Autodesk Inventor part; units mm, degrees
ref_plane "YZ Plane" through (0, 0, 0) normal (1, 0, 0) x (0, 1, 0)
ref_plane "XZ Plane" through (0, 0, 0) normal (0, 1, 0) x (-1, 0, 0)
ref_plane "XY Plane" through (0, 0, 0) normal (0, 0, 1) x (1, 0, 0)
sketch "Sketch_1" plane through (0, 0, 0) normal (0, 0, 1) x (1, 0, 0)
  line L0 (5, 0) -> (-0.8, 0)
  line L1 (-0.8, 0) -> (-0.8, 2)
  line L2 (-0.8, 2) -> (-0.2226, 3)
  line L3 (-0.2226, 3) -> (0, 3)
  line L4 (0, 3) -> (0, 1.4467)
  arc A0 (0, 1.4467) -> (0.1, 1.3467) centre (0.1, 1.4467) ccw
  line L5 (0.1, 1.3467) -> (0.9, 1.3467)
  line L6 (0.9, 1.3467) -> (1.4, 1.5)
  line L7 (1.4, 1.5) -> (4.6935, 1.5)
  line L8 (4.6935, 1.5) -> (5, 1.1935)
  line L9 (5, 1.1935) -> (5, 0)
  line L10 (5, 0) -> (-0.8, 0)
revolve "Revolution1" add sketch "Sketch_1" angle 360 about axis through (5, 0, 0) along (1, 0, 0)
thread "Thread1"
sketch "Sketch2" plane through (-0.8, 0, 0) normal (-1, 0, 0) x (0, 0, 1)
  point P0 (0, 0)
hole "Hole1" at (-0.8, 0, 0) direction (1, 0, 0) diameter 1.5 depth 2 tip angle 120
sketch "Sketch_3" plane through (-0.8, 0, 0) normal (1, 0, 0) x (0, 0, -1)
  line L0 (-0.75, -0.433) -> (0, -0.866)
  line L1 (0, -0.866) -> (0.75, -0.433)
  line L2 (0.75, -0.433) -> (0.75, 0.433)
  line L3 (0.75, 0.433) -> (0, 0.866)
  line L4 (0, 0.866) -> (-0.75, 0.433)
  line L5 (-0.75, 0.433) -> (-0.75, -0.433)
extrude "Extrusion1" cut sketch "Sketch_3" along normal blind 2
properties part number "CBSTSR3-5"
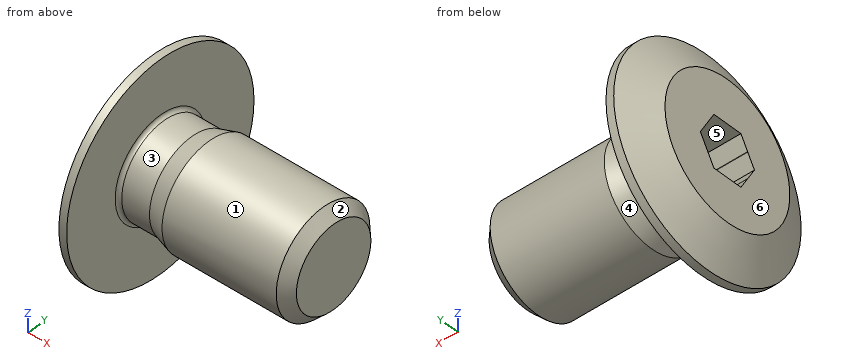
Work out the finished part from the listing and answer in its coordinate system (mm). Face numbers are marked on the shaded views. A direction names the side the tool comes from. Round coordinates to 2 decimals unless told otherwise and drop trailing zeros. Loops run counter-clockwise (first coordinate to the right, second up) from the corner with the lowest first, then second, coordinate; pieces in that order, holes last. Notation, with made-up numbers: (-7.5, -14) -> (43.5, -14) arc R11 ccw to (43.5, -7) -> close; hole circle Ø5 at (-22.75, -11.75). An arc over 180 degrees is marked (long way). Use one line per item in the form item = value.
(1) A tool of negligible diameter and unlimited length cuts with its end or side. For the marked faces 4, 5 and 6, from which of +Z, -Z, +X, -X, +Y, -Y can it reach the whole face along a straight path? Write none if from no direction.
Answer list:
face_4 = none
face_5 = -X
face_6 = +Z, -Z, -X, +Y, -Y
(2) For a pull along X with two mould halves and no side action, classify the marked faces 1, 2 and 3 as released by +X, released by -X, zero draft, split by the parting line, or undercut.
Answer list:
face_1 = zero draft
face_2 = released by +X
face_3 = undercut
(3) A flat-ended cylindrical pin translates along its axis: P1, Ø1.5, axis at x = 2, z = -1, coming from the +Y side. Find the tip coordinate at first contact, or state that the pin passes through.
Answer list:
P1 = 1.48
(4) Straight lines are drawn through the part: line 1 (X direction, y = 1.25, z = 1.4); line 2 (Y direction, x = 0.55, z = -0.05); line 3 (Z direction, x = 0.6, y = -0.75). For each, find the intervals that lie inside material, in ascending order.
Answer list:
line_1 = -0.8 to 0
line_2 = -1.35 to -0.84, 0.84 to 1.35
line_3 = -1.12 to -0.2, 0.2 to 1.12
(5) Find section B-B on x = 1.9. Give the vertices of the cut face in (y, z), then the cut area to 3 significant figures.
Answer list:
outline = circle Ø3 at (0, 0)
area = 7.07 mm2
